Answer from the drawing. Dimensions are ordinates in mm from the lowest x, y and z of the part. Coordinates: 2 decimals unless noted, no trailing zeros. Order: outer loops, then holes, each group sorted by start corner. A loop starts at its lowest first (then second) coordinate and runs counter-clockwise, first axis right, second up. Notation, with made-up numbers: (-36.5, 46) -> (-1.5, 46) arc R31 cw to (-1.5, 70) -> close; hole circle Ø9 at (-7.75, -12). An arc over 180 degrees is marked (long way). Use CSV: the item, a comma, the result in double quotes.
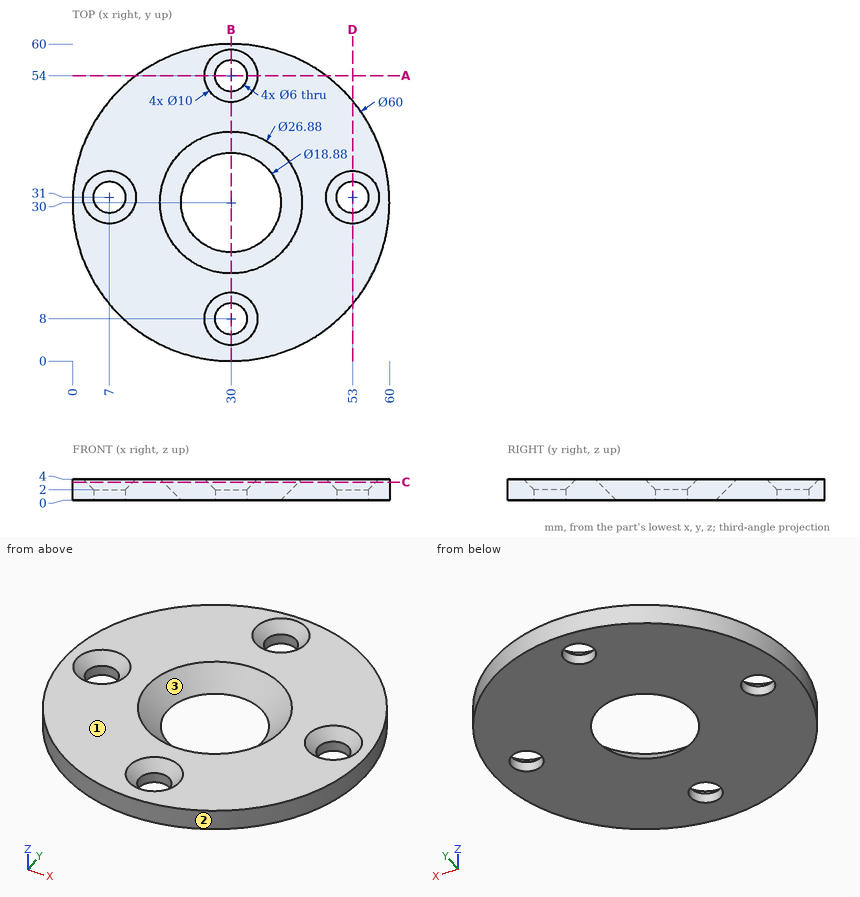
Item 1: Straight lines are drawn through the part: line 1 along X through (y, z) = (54, 0.6); line 2 along Y through (x, z) = (32.5, 1.3); line 3 along Y through (x, z) = (30, 0.9). For each, find the intervals that lie inside material, in ascending order.
Return value:
line 1,"x = 12 to 27, 33 to 48"
line 2,"y = 0.1 to 6.34, 9.66 to 19.56, 40.44 to 52.34, 55.66 to 59.9"
line 3,"y = 0 to 5, 11 to 19.66, 40.34 to 51, 57 to 60"
Item 2: Find section A-A, the plane y = 54. Give the vertices of the cut face in (x, z).
Return value:
outline,"(12, 0) -> (27, 0) -> (27, 2) -> (25, 4) -> (12, 4) -> close; (33, 0) -> (48, 0) -> (48, 4) -> (35, 4) -> (33, 2) -> close"
Item 3: Find section D-D, the plane x = 53. Give the vertices of the cut face in (y, z), then the cut area to 3 significant figures.
Return value:
outline,"(10.74, 0) -> (28, 0) -> (28, 2) -> (26, 4) -> (10.74, 4) -> close; (34, 0) -> (49.26, 0) -> (49.26, 4) -> (36, 4) -> (34, 2) -> close"
area,"126 mm^2"
Item 4: The mould has two halves that part along X. Classify the marked faces 1, 2 and 3: +X half, -X half, draft (parallel to the pull), parting line (faces both ways), or undercut.
Return value:
face 1,"draft"
face 2,"parting line"
face 3,"undercut"
Item 5: Each of these flat-tipped pins is pushed along its axis until it touches: P1, Ø1.5, axis at x = 49, z = 1.5, coming from the -Y side; P2, Ø2, axis at x = 22, z = 2, coming from the -Y side; P3, Ø5, axis at x = 30, y = 54, coming from the +Z side; P4, Ø1, axis at x = 42, z = 2, coming from the -Y side. Where does it stop, or does it pass through?
Return value:
P1,"stops at y = 6.19"
P2,"stops at y = 0.83"
P3,"passes through"
P4,"stops at y = 2.29"
Item 6: Find section B-B, the plane x = 30. Give the vertices of the cut face in (y, z).
Return value:
outline,"(0, 0) -> (5, 0) -> (5, 2) -> (3, 4) -> (0, 4) -> close; (11, 0) -> (20.56, 0) -> (16.56, 4) -> (13, 4) -> (11, 2) -> close; (39.44, 0) -> (51, 0) -> (51, 2) -> (49, 4) -> (43.44, 4) -> close; (57, 0) -> (60, 0) -> (60, 4) -> (59, 4) -> (57, 2) -> close"
Item 7: Find section C-C, the plane z = 3.4. Give the vertices of the cut face in (x, y).
Return value:
outline,"circle Ø60 at (30, 30); hole circle Ø8.8 at (7, 31); hole circle Ø25.68 at (30, 30); hole circle Ø8.8 at (30, 8); hole circle Ø8.8 at (30, 54); hole circle Ø8.8 at (53, 31)"
